Check sheet for the modelled part. Datum: model origin and axes. Units: mm. A direction names the side the tool comes from. Round coordinates to 2 decimals unless told otherwise and drop trailing zeros. Loops run counter-clockwise (first coordinate to the right, second up) from the corner with the lowest first, then second, coordinate; pieces in that order, holes last. Notation, with made-up numbers: (33.25, 41.25) - (59.25, 41.25) arc R12 cw to (59.25, 64.25) - close; hole circle Ø9 at (52, 21). An arc over 180 degrees is marked (long way). Put each result on its own line as item: value.
```python
from build123d import *

# Parameters (mm, degrees)
SKETCH1_W               = 114.3
SKETCH1_H               = 76.2
BASE_EXTRUDE_DEPTH      = 19.05
F_1_2_20_TAPPED_HOLE1_D = 12.7
CUT_EXTRUDE1_DEPTH      = 12.7
CUT_EXTRUDE2_DEPTH      = 12.7
SKETCH7_W               = 6.35
SKETCH7_H               = 76.2
CUT_EXTRUDE3_DEPTH      = 1
CUT_EXTRUDE3_DEPTH_BACK = 20.05
SKETCH8_W               = 6.35
SKETCH8_H               = 76.2
CUT_EXTRUDE4_DEPTH      = 1
CUT_EXTRUDE4_DEPTH_BACK = 20.05
CUT_EXTRUDE5_DEPTH      = 1
CUT_EXTRUDE5_DEPTH_BACK = 20.05


with BuildPart() as part:
    # Sketch1 → Base-Extrude (new body)
    with BuildSketch(Plane(origin=(0, 0, 0), x_dir=(1, 0, 0), z_dir=(0, 1, 0))):
        with Locations((57.15, 38.1)):
            Rectangle(SKETCH1_W, SKETCH1_H)
        with BuildLine():
            Line((96.012, 63.5), (96.012, 38.1))
            ThreePointArc((96.012, 38.1), (88.9, 30.988), (81.788, 38.1))
            Line((81.788, 38.1), (81.788, 63.5))
            ThreePointArc((81.788, 63.5), (88.9, 70.612), (96.012, 63.5))
        make_face(mode=Mode.SUBTRACT)
        with BuildLine():
            Line((18.288, 63.5), (18.288, 38.1))
            ThreePointArc((18.288, 38.1), (25.4, 30.988), (32.512, 38.1))
            Line((32.512, 38.1), (32.512, 63.5))
            ThreePointArc((32.512, 63.5), (25.4, 70.612), (18.288, 63.5))
        make_face(mode=Mode.SUBTRACT)
    extrude(amount=BASE_EXTRUDE_DEPTH)

    # 1/2-20 Tapped Hole1 (through all)
    with Locations(Plane(origin=(0, 19.05, 0), x_dir=(-1, 0, 0), z_dir=(0, 1, 0))):
        with Locations((-25.4, -19.05), (-88.9, -19.05)):
            Hole(F_1_2_20_TAPPED_HOLE1_D / 2)

    # Sketch4 → Cut-Extrude1 (cut)
    with BuildSketch(Plane.XZ):
        with BuildLine():
            Line((15.0749, -63.5), (15.0749, -38.1))
            ThreePointArc((15.0749, -38.1), (25.4, -27.7749), (35.7251, -38.1))
            Line((35.7251, -38.1), (35.7251, -63.5))
            ThreePointArc((35.7251, -63.5), (25.4, -73.8251), (15.0749, -63.5))
        make_face()
    extrude(amount=-CUT_EXTRUDE1_DEPTH, mode=Mode.SUBTRACT)

    # Sketch5 → Cut-Extrude2 (cut)
    with BuildSketch(Plane.XZ):
        with BuildLine():
            Line((99.2251, -38.1), (99.2251, -63.5))
            ThreePointArc((99.2251, -63.5), (88.9, -73.8251), (78.5749, -63.5))
            Line((78.5749, -63.5), (78.5749, -38.1))
            ThreePointArc((78.5749, -38.1), (88.9, -27.7749), (99.2251, -38.1))
        make_face()
    extrude(amount=-CUT_EXTRUDE2_DEPTH, mode=Mode.SUBTRACT)

    # Sketch7 → Cut-Extrude3 (cut, two sides)
    with BuildSketch(Plane.XZ) as cut_extrude3_sk:
        with Locations((111.125, -38.1)):
            Rectangle(SKETCH7_W, SKETCH7_H)
    extrude(amount=CUT_EXTRUDE3_DEPTH, mode=Mode.SUBTRACT)
    extrude(cut_extrude3_sk.sketch, amount=-CUT_EXTRUDE3_DEPTH_BACK, mode=Mode.SUBTRACT)

    # Sketch8 → Cut-Extrude4 (cut, two sides)
    with BuildSketch(Plane.XZ) as cut_extrude4_sk:
        with Locations((3.175, -38.1)):
            Rectangle(SKETCH8_W, SKETCH8_H)
    extrude(amount=CUT_EXTRUDE4_DEPTH, mode=Mode.SUBTRACT)
    extrude(cut_extrude4_sk.sketch, amount=-CUT_EXTRUDE4_DEPTH_BACK, mode=Mode.SUBTRACT)

    # Sketch9 → Cut-Extrude5 (cut, two sides)
    with BuildSketch(Plane.XZ) as cut_extrude5_sk:
        Polygon((351.091008834, -57.15), (107.95, -57.15), (6.35, -57.15), (-236.791008834, -57.15), (-236.791008834, -543.432017667), (351.091008834, -543.432017667), align=None)
    extrude(amount=CUT_EXTRUDE5_DEPTH, mode=Mode.SUBTRACT)
    extrude(cut_extrude5_sk.sketch, amount=-CUT_EXTRUDE5_DEPTH_BACK, mode=Mode.SUBTRACT)


solid = part.part
```
Item 1: Section check B-B on x = 25.4. Enter the section's corners in (y, z), then the cut area to 3 significant figures.
Filled sheet:
outline: (0, -27.77) - (12.7, -27.77) - (12.7, -30.99) - (19.05, -30.99) - (19.05, -25.4) - (0, -25.4) - close; (0, -12.7) - (19.05, -12.7) - (19.05, 0) - (0, 0) - close
area: 308 mm²
Item 2: Thickness scan on line 1 (X direction, y = 17, z = -53.5); line 2 (X direction, y = 12, z = -52.5); line 3 (Z direction, x = 88.9, y = 8.5). Record the ranges inside material, lowest first. Write a range as from..to.
Filled sheet:
line 1: 6.35..18.29, 32.51..81.79, 96.01..107.95
line 2: 6.35..15.07, 35.73..78.57, 99.23..107.95
line 3: -27.77..-25.4, -12.7..0
Item 3: Section check C-C on y = 11.75. Enter the section's corners in (x, z), then the cut area to 3 significant figures.
Filled sheet:
outline: (6.35, -57.15) - (15.07, -57.15) - (15.07, -38.1) arc R10.33 cw to (35.73, -38.1) - (35.73, -57.15) - (78.57, -57.15) - (78.57, -38.1) arc R10.33 cw to (99.23, -38.1) - (99.23, -57.15) - (107.95, -57.15) - (107.95, 0) - (6.35, 0) - close; hole circle Ø12.7 at (25.4, -19.05); hole circle Ø12.7 at (88.9, -19.05)
area: 4,430 mm²
Item 4: Release check for a two-part mould opening along X. For faces 1 (the cylindrical face through (88.673, 6.261, -27.777)), 2 (the flat face through (107.95, 9, -29)), 3 (the flat face through (57, 9, -57.15)) record: +X half, -X half, draft (parallel to the pull), parting line (faces both ways), or undercut.
Filled sheet:
face 1: undercut
face 2: +X half
face 3: draft
Item 5: Section check A-A on z = -19.05. Enter the section's corners in (x, y), then the cut area to 3 significant figures.
Filled sheet:
outline: (6.35, 0) - (19.05, 0) - (19.05, 19.05) - (6.35, 19.05) - close; (31.75, 0) - (82.55, 0) - (82.55, 19.05) - (31.75, 19.05) - close; (95.25, 0) - (107.95, 0) - (107.95, 19.05) - (95.25, 19.05) - close
area: 1,450 mm²
Item 6: Go/stop test with flat-tipped pins: pin 1 (11.5 mm diameter, centred on x = 88.9, z = -19.05, fed in from +Y); pin 2 (8 mm diameter, centred on x = 81.5, z = -48, fed in from -Y); pin 3 (6 mm diameter, centred on x = 85, z = -35.5, fed in from -Y). Record where each tip stops, or that it passes through.
Filled sheet:
pin 1: through
pin 2: y = 0
pin 3: y = 12.7
Item 7: Section check D-D on z = -32. Enter the section's corners in (x, y).
Filled sheet:
outline: (6.35, 0) - (17.07, 0) - (17.07, 12.7) - (21.74, 12.7) - (21.74, 19.05) - (6.35, 19.05) - close; (29.06, 12.7) - (33.73, 12.7) - (33.73, 0) - (80.57, 0) - (80.57, 12.7) - (85.24, 12.7) - (85.24, 19.05) - (29.06, 19.05) - close; (92.56, 12.7) - (97.23, 12.7) - (97.23, 0) - (107.95, 0) - (107.95, 19.05) - (92.56, 19.05) - close
Item 8: Tool access check on faces 4 (the flat face through (99.225, 6, -47)), 5 (the flat face through (56, 19.05, -29)), 6 (the flat face through (18.288, 16, -48)). Record the directions out of +Z, -Z, +X, -X, +Y, -Y that give a thin tool (end or side, any length) a straight path to the whole face; none if there is none.
Filled sheet:
face 4: -Z, -Y
face 5: +Z, -Z, +X, -X, +Y
face 6: -Z, +Y, -Y
